```python
from build123d import *

# Parameters (mm, degrees)
SKETCH1_R           = 101.6
SKETCH1_R_2         = 25.4
BOSS_EXTRUDE1_DEPTH = 190.5
SKETCH2_R           = 101.6
BOSS_EXTRUDE2_DEPTH = 101.6
BOSS_EXTRUDE2_TAPER = 37
SKETCH3_R           = 101.6
BOSS_EXTRUDE3_DEPTH = 101.6
BOSS_EXTRUDE3_TAPER = 37
SKETCH4_R           = 25.03890851
CUT_EXTRUDE1_DEPTH  = 453.39
SKETCH5_R           = 25.4
CUT_EXTRUDE3_DEPTH  = 351.79


with BuildPart() as part:
    # Sketch1 → Boss-Extrude1 (new body)
    with BuildSketch(Plane(origin=(0, 0, 0), x_dir=(0, 0, -1), z_dir=(1, 0, 0))):
        Circle(SKETCH1_R)
        Circle(SKETCH1_R_2, mode=Mode.SUBTRACT)
    extrude(amount=BOSS_EXTRUDE1_DEPTH)

    # Sketch2 → Boss-Extrude2 (add)
    with BuildSketch(Plane(origin=(190.5, 0, 0), x_dir=(0, 0, -1), z_dir=(1, 0, 0))):
        Circle(SKETCH2_R)
    extrude(amount=BOSS_EXTRUDE2_DEPTH, taper=BOSS_EXTRUDE2_TAPER)

    # Sketch3 → Boss-Extrude3 (add)
    with BuildSketch(Plane.ZY):
        Circle(SKETCH3_R)
    extrude(amount=BOSS_EXTRUDE3_DEPTH, taper=BOSS_EXTRUDE3_TAPER)

    # Sketch4 → Cut-Extrude1 (cut)
    with BuildSketch(Plane.ZY.offset(101.6)):
        with Locations(Location((0, 0, 0), (0, 0, 180))):
            Circle(SKETCH4_R)
    extrude(amount=-CUT_EXTRUDE1_DEPTH, mode=Mode.SUBTRACT)

    # Sketch5 → Cut-Extrude3 (cut)
    with BuildSketch(Plane.XY.offset(254)):
        with Locations((95.115505382, 0)):
            Circle(SKETCH5_R)
    extrude(amount=-CUT_EXTRUDE3_DEPTH, mode=Mode.SUBTRACT)


solid = part.part
```
Design review of the part built by this model. Coordinates are the model's own, in mm. A direction names the side the tool comes from. Coordinates: 2 decimals unless noted, no trailing zeros. Order: outer loops, then holes, each group sorted by start corner. A loop starts at its lowest first (then second) coordinate and runs counter-clockwise, first axis right, second up.
1) Mouldability with a two-part tool opening along Y and no side actions: class faces 4 (the cylindrical face through (36.324, 7.629, -24.227)), 5 (the conical face through (-85.38, -33.06, 17.19)) as +Y half, -Y half, draft (parallel to the pull), parting line (faces both ways), or undercut.
2) Clearance check with flat-ended pins moving along their axes: pin 1 (12 mm diameter, centred on x = 185.5, z = 24, fed in from +Y); pin 2 (6 mm diameter, centred on x = 188.5, z = 10, fed in from -Y); pin 3 (10 mm diameter, centred on y = -20.5, z = -67.5, fed in from -X). State where each tip first meets the part, or that it passes through.
3) Take a section at C-C, the plane x = -74. Give the boundary of the cut face in (y, z).
4) Take a section at A-A, the plane x = 76.5. Give the boundary of the cut face in (y, z).
5) For faces 1 (the flat face through (0, 11.4, 22.5)), 2 (the cylindrical face through (119.343, 7.629, 62.8)), 3 (the cylindrical face through (-51.511, 24.443, 5.428)), list the 3-axis set-ups (+Z, -Z, +X, -X, +Y, -Y) from which the entire face can be reached by the end or side of a thin tool; tool diameter is ignored.
6) Take a section at B-B, the plane y = 0. State how many separate pieces and enclosed holes the cut face has, and give its area (3 significant figures).
7) Wall thickness on line 1 along Z through (x, y) = (162.5, 0); line 2 along Y through (x, z) = (233, 0); line 3 along Z through (x, y) = (-49.5, -17): over which ranges is each line inside the solid? List them lowest first.
Returned:
1. face 4: undercut
1. face 5: parting line
2. pin 1: stops at y = 99.99
2. pin 2: stops at y = -101.36
2. pin 3: stops at x = -47.85
3. outline: circle Ø91.67 at (0, 0); hole circle Ø50.08 at (0, 0)
4. outline: (-17.28, -97.79) - (-17.28, -18.62) arc R25.4 cw to (-17.28, 18.62) - (-17.28, 100.12) arc R101.6 ccw (long way) to (17.28, 100.12) - (17.28, 18.62) arc R25.4 cw to (17.28, -18.62) - (17.28, -97.79) - close
5. face 1: none
5. face 2: +Z
5. face 3: +X, -X
6. separate pieces: 3
6. enclosed holes: 0
6. area: 37,000 mm2
7. line 1: z = -101.6 to -25.4, 25.4 to 101.6
7. line 2: y = -69.57 to -25.04, 25.04 to 69.57
7. line 3: z = -62.01 to -18.38, 18.38 to 62.01
